Autodesk Inventor part; units mm, degrees
ref_plane "YZ Plane" through (0, 0, 0) normal (1, 0, 0) x (0, 1, 0)
ref_plane "XZ Plane" through (0, 0, 0) normal (0, 1, 0) x (-1, 0, 0)
ref_plane "XY Plane" through (0, 0, 0) normal (0, 0, 1) x (1, 0, 0)
sketch "Sketch1" plane through (0, 0, 0) normal (0, 1, 0) x (-1, 0, 0)
  line L0 (-127, 19.05) -> (-127, -19.05)
  line L1 (127, -19.05) -> (127, 19.05)
  line L2 (0, -127) -> (19.05, -127)
  line L3 (19.05, -127) -> (19.05, -19.05)
  line L4 (19.05, 0) -> (0, 0)
  line L5 (0, -127) -> (-19.05, -127)
  line L6 (-19.05, -127) -> (-19.05, -19.05)
  line L7 (-19.05, 0) -> (0, 0)
  line L8 (0, 0) -> (0, -127)
  line L9 (19.05, 0) -> (0, 0)
  line L10 (-19.05, 0) -> (-19.05, 127)
  line L11 (-19.05, 127) -> (19.05, 127)
  line L12 (19.05, 127) -> (19.05, 19.05)
  line L13 (-127, -19.05) -> (-19.05, -19.05)
  line L14 (19.05, -19.05) -> (127, -19.05)
  line L15 (127, 19.05) -> (19.05, 19.05)
  line L16 (-19.05, 19.05) -> (-127, 19.05)
  point P0 (127, 0)
  point P1 (-127, 0)
  point P2 (0, 19.05)
  point P3 (0, -19.05)
  dimension "d7" = 127
  dimension "d8" = 19.05
  dimension "d9" = 127
extrude "Extrusion1" add sketch "Sketch1" along normal blind 38.1
sketch "Sketch2" plane through (0, 38.1, 0) normal (0, 1, 0) x (1, 0, 0)
  line L0 (-19.05, -127) -> (19.05, -127)
  line L1 (-19.05, -127) -> (19.05, -127)
  line L2 (19.05, -127) -> (19.05, -88.9)
  line L3 (19.05, -88.9) -> (-19.05, -88.9)
  line L4 (-19.05, -88.9) -> (-19.05, -127)
  line L5 (-19.05, 127) -> (-19.05, 19.05)
  line L6 (19.05, 19.05) -> (19.05, 127)
  line L7 (-19.05, 127) -> (19.05, 127)
  line L8 (19.05, 127) -> (19.05, 88.9)
  line L9 (19.05, 88.9) -> (-19.05, 88.9)
  line L10 (-19.05, 88.9) -> (-19.05, 127)
  line L11 (-127, -19.05) -> (-19.05, -19.05)
  line L12 (-19.05, 19.05) -> (-127, 19.05)
  line L13 (-127, -19.05) -> (-88.9, -19.05)
  line L14 (-88.9, -19.05) -> (-88.9, 19.05)
  line L15 (-88.9, 19.05) -> (-127, 19.05)
  line L16 (-127, 19.05) -> (-127, -19.05)
  line L17 (127, -19.05) -> (127, 19.05)
  line L18 (127, 19.05) -> (19.05, 19.05)
  line L19 (127, -19.05) -> (88.9, -19.05)
  line L20 (88.9, -19.05) -> (88.9, 19.05)
  line L21 (88.9, 19.05) -> (127, 19.05)
  line L22 (127, 19.05) -> (127, -19.05)
  point P0 (0, 0)
  point P1 (-19.05, 88.9)
  dimension "d12" = 38.1
  dimension "d13" = 38.1
  dimension "d14" = 38.1
  dimension "d15" = 38.1
  dimension "d16" = 38.1
extrude "Extrusion2" add sketch "Sketch2" along normal blind 19.05
sketch "Sketch3" plane through (0, 0, 0) normal (0, -1, 0) x (1, 0, 0)
  circle A0 centre (0, 0) radius 38.1
  dimension "d19" = 76.2
extrude "Extrusion3" add sketch "Sketch3" along normal blind 25.4
sketch "Sketch4" plane through (0, -25.4, 0) normal (0, -1, 0) x (1, 0, 0)
  circle A0 centre (0, 0) radius 34.925
  dimension "d22" = 69.85
extrude "Extrusion4" add sketch "Sketch4" along normal blind 190.5
sketch "Sketch5" plane through (0, -215.9, 0) normal (0, -1, 0) x (1, 0, 0)
  circle A0 centre (0, 0) radius 34.925
  line L0 (24.9762, 24.412) -> (-24.9888, 24.412)
  line L1 (-24.9888, 24.412) -> (-24.9888, -24.3991)
  line L2 (-24.9888, -24.3991) -> (24.9762, -24.3991)
  line L3 (24.9762, -24.3991) -> (24.9762, 24.412)
  point P0 (-24.9762, 24.412)
  point P1 (-24.9888, 24.3991)
extrude "Extrusion5" add sketch "Sketch5" along normal blind 50.8 contours L3 L2 L1 A0 L0
sketch "Sketch6" plane through (24.9762, -215.9, -24.3991) normal (0, 0, -1) x (-1, 0, 0)
  line L0 (11.8903, -39.6018) -> (38.7164, -39.6018)
  line L1 (38.7164, -39.6018) -> (38.7164, -13.4301)
  line L2 (38.7164, -13.4301) -> (11.8903, -13.4301)
  line L3 (11.8903, -13.4301) -> (11.8903, -39.6018)
  point P0 (24.9762, 215.9)
extrude "Extrusion6" add sketch "Sketch6" along normal blind 19.05
fillet "Fillet1" radius 3.175 7 edges at (-0.3271, -255.5018, -43.4491) (13.0859, -255.5018, -33.9241) (13.0859, -242.416, -43.4491) (13.0859, -229.3301, -33.9241) (-0.3271, -229.3301, -43.4491) (-13.7402, -229.3301, -33.9241) (-13.7402, -242.416, -43.4491)
fillet "Fillet2" radius 3.175 2 edges at (-12.8102, -254.5719, -42.5191) (-13.7402, -255.5018, -32.3366)
sketch "Sketch7" plane through (0, -266.7, 0) normal (0, -1, 0) x (1, 0, 0)
  circle A0 centre (0, 0) radius 22.225
  dimension "d31" = 44.45
extrude "Extrusion7" add sketch "Sketch7" along normal blind 254
sketch "Sketch8" plane through (0, -520.7, 0) normal (0, -1, 0) x (1, 0, 0)
  point P0 (0, 0)
properties part number "stand"
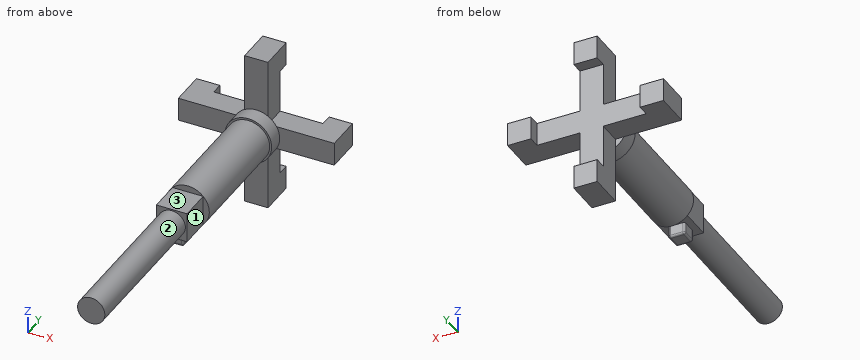
CAD build for the part. Positions are in the model's coordinates, mm. Face numbers are marked on the shaded views. A direction names the side the tool comes from. Round coordinates to 2 decimals unless told otherwise and drop trailing zeros. Order: outer loops, then holes, each group sorted by start corner. A loop starts at its lowest first (then second) coordinate and runs counter-clockwise, first axis right, second up.
Q1. Slice it at D-D (z = 77). Write the cut outline in (x, y), and give its area (3 significant figures).
Q2. Slice it at C-C (y = -280). Write the cut outline in (x, z) (3 decimals).
Q3. Which spindle directions (+Z, -Z, +X, -X, +Y, -Y) get a long thin tool onto all of the face, cutting with end or side? Do the marked faces 1, 2 and 3. Say none if no direction does.
Q4. Slice it at A-A (z = 0). Write the cut outline in (x, y) (3 decimals).
Q5. Drop flat-ended pins along their axis: pin 1 (5 mm diameter, centred on x = 2, z = -54, fed in from -Y); pin 2 (5.5 mm diameter, centred on x = -4, z = 28, fed in from -Y); pin 3 (17 mm diameter, centred on x = -96, y = 25, fed in from -Z); pin 4 (12 mm diameter, centred on x = -33, y = -237, fed in from -Z). Give the stop position or say it passes through.
Q6. Wall check: L1, parallel to Y at x = 12, z = -64; L2, parallel to X at y = 21, z = 85.5; L3, parallel to Y at x = -20, z = -15.5. Give the ranges that are in metal, low to high.
Results below:
1. outline: (-19.05, 0) - (19.05, 0) - (19.05, 38.1) - (-19.05, 38.1) - close
1. area: 1,450 mm2
2. outline: circle Ø44.45 at (0, 0)
3. face 1: +Z, -Z, +X, -Y
3. face 2: -Y
3. face 3: +Z, +X, -X, -Y
4. outline: (-127, 0) - (-38.1, 0) - (-38.1, -25.4) - (-34.925, -25.4) - (-34.925, -215.9) - (-24.989, -215.9) - (-24.989, -266.7) - (-22.225, -266.7) - (-22.225, -520.7) - (22.225, -520.7) - (22.225, -266.7) - (24.976, -266.7) - (24.976, -215.9) - (34.925, -215.9) - (34.925, -25.4) - (38.1, -25.4) - (38.1, 0) - (127, 0) - (127, 57.15) - (88.9, 57.15) - (88.9, 38.1) - (-88.9, 38.1) - (-88.9, 57.15) - (-127, 57.15) - close
5. pin 1: stops at y = 0
5. pin 2: stops at y = -215.9
5. pin 3: stops at z = -19.05
5. pin 4: passes through
6. L1: y = 0 to 38.1
6. L2: x = -19.05 to 19.05
6. L3: y = -266.7 to 38.1
